Work out the finished part from the listing and answer in its coordinate system (mm). A direction names the side the tool comes from. Coordinates: 2 decimals unless noted, no trailing zeros. Write each loop counter-clockwise with the first axis right and the second up, starting at its lowest first coordinate (ties: lowest second). Pieces come first, ordered by that corner, then holes. Notation, with made-up numbers: M 29,75.25 L 45,75.25 A19 cw 45,103.25 Z; hole C -12.75,63 d7. An arc over 180 degrees is marked long. Use CSV: the item, a comma, the result in double quotes.
from build123d import *

# Parameters (mm, degrees)
SKETCH1_R           = 161.925
BOSS_EXTRUDE1_DEPTH = 797.56
SKETCH2_R           = 84.201
BOSS_EXTRUDE2_DEPTH = 405.13
SKETCH3_R           = 146.7485
CUT_EXTRUDE1_DEPTH  = 798.5600001
CUT_EXTRUDE2_REACH  = 569.055
SKETCH4_R           = 76.6953


with BuildPart() as part:
    # Sketch1 → Boss-Extrude1 (new body)
    with BuildSketch(Plane(origin=(0, 0, 0), x_dir=(1, 0, 0), z_dir=(0, 1, 0))):
        Circle(SKETCH1_R)
    extrude(amount=BOSS_EXTRUDE1_DEPTH)

    # Sketch2 → Boss-Extrude2 (add)
    with BuildSketch(Plane(origin=(0, 0, 0), x_dir=(0, 0, -1), z_dir=(1, 0, 0))):
        with Locations((0, 398.78)):
            Circle(SKETCH2_R)
    extrude(amount=BOSS_EXTRUDE2_DEPTH)

    # Sketch3 → Cut-Extrude1 (cut, through all)
    with BuildSketch(Plane.XZ):
        Circle(SKETCH3_R)
    extrude(amount=-CUT_EXTRUDE1_DEPTH, mode=Mode.SUBTRACT)

    # Sketch4 → Cut-Extrude2 (cut, up to next)
    with BuildSketch(Plane(origin=(405.13, 0, 0), x_dir=(0, 0, -1), z_dir=(1, 0, 0)), mode=Mode.PRIVATE) as cut_extrude2_sk1:
        with Locations((0, 398.78)):
            Circle(SKETCH4_R)
    cut_extrude2_tool1 = extrude(cut_extrude2_sk1.sketch, amount=-CUT_EXTRUDE2_REACH, mode=Mode.PRIVATE) & part.part
    add(cut_extrude2_tool1.solids().sort_by_distance((405.13, 398.78, 0))[0], mode=Mode.SUBTRACT)


solid = part.part
Item 1: For a pull along Y with two mould halves and no side action, classify faces 3 (the face through (267.081, 421.817, -73.154)), 4 (the face through (405.13, 417.9, -74.5)), 5 (the face through (-145, 0, -25)) as released by +Y, released by -Y, zero draft, split by the parting line, or undercut.
Answer:
face 3,"undercut"
face 4,"zero draft"
face 5,"released by -Y"
Item 2: The part is cut by section B-B (x = 0). Write down the section's boundary in (y, z) (1 decimal).
Answer:
outline,"M 0,-161.9 L 797.6,-161.9 L 797.6,-146.7 L 0,-146.7 Z; M 0,146.7 L 797.6,146.7 L 797.6,161.9 L 0,161.9 Z"
Item 3: Consider probe 1 along Z at (x, y) = (341.5, 398.78); probe 2 along Y at (x, z) = (272, 0); probe 3 along X at (y, z) = (709, -18.5). Determine where each line is inside the solid, lowest interval first.
Answer:
probe 1,"z = -84.2 to -76.7, 76.7 to 84.2"
probe 2,"y = 314.58 to 322.08, 475.48 to 482.98"
probe 3,"x = -160.86 to -145.58, 145.58 to 160.86"
Item 4: Given pin 1 (10 mm diameter, centred on x = 208, z = -58.5, fed in from +Y); pin 2 (1 mm diameter, centred on x = 85, y = 253, fed in from -Z); pin 3 (1.5 mm diameter, centred on x = 242, z = 74, fed in from +Y), each flat-ended and moving along its own axis, determine where each tip first touches the part or whether it passes through.
Answer:
pin 1,"stops at y = 463.8"
pin 2,"stops at z = -138.13"
pin 3,"stops at y = 440.3"
Item 5: The part is cut by section A-A (z = 0). Write down the section's boundary in (x, y) (1 decimal), then the cut area to 3 significant figures.
Answer:
outline,"M -161.9,0 L -146.7,0 L -146.7,797.6 L -161.9,797.6 Z; M 146.7,0 L 161.9,0 L 161.9,314.6 L 405.1,314.6 L 405.1,322.1 L 146.7,322.1 Z; M 146.7,475.5 L 405.1,475.5 L 405.1,483 L 161.9,483 L 161.9,797.6 L 146.7,797.6 Z"
area,"25,500 mm2"
Item 6: The part is cut by section D-D (z = -94). Write down the section's boundary in (x, y).
Answer:
outline,"M -131.85,0 L -112.69,0 L -112.69,797.56 L -131.85,797.56 Z; M 112.69,0 L 131.85,0 L 131.85,797.56 L 112.69,797.56 Z"
Item 7: A tool of negligible diameter and unlimited length cuts with its end or side. For faces 1 (the face through (-146.607, 393.197, 6.452)), 2 (the face through (269.85, 402.48, 84.12)), from which of +Z, -Z, +X, -X, +Y, -Y can it reach the whole face along a straight path? Write none if from no direction.
Answer:
face 1,"+Y, -Y"
face 2,"+X"
